from build123d import *

# Parameters (mm, degrees)
F1_DEPTH = 3.81
F2_DEPTH = 25.4
F4_DEPTH = 25.4


with BuildPart() as f1:
    # F0 (on Top) → F1 (new body)
    with BuildSketch(Plane.XY):
        Polygon((6.5642443103, 3.7926732977), (-0.0024292689, 7.5811389783), (-6.5666735793, 3.7884656805), (-6.5642443103, -3.7926732977), (0.0024292689, -7.5811389783), (6.5666735793, -3.7884656805), align=None)
        Polygon((-4.0262038002, 2.3228099792), (-0.00148945, 4.6481997614), (4.0247143502, 2.3253897822), (4.0262038002, -2.3228099792), (0.00148945, -4.6481997614), (-4.0247143502, -2.3253897822), align=None, mode=Mode.SUBTRACT)
    extrude(amount=F1_DEPTH)

    # F2 (add): a face of the model
    f2_faces = [f1.faces().sort_by_distance(p)[0] for p in [
        (3.2845514241, -5.6848023294, 1.905),
    ]]
    extrude(f2_faces, amount=F2_DEPTH)

    # F3 (on face) → F4 (cut)
    with BuildSketch(Plane.XY.offset(3.81)):
        Polygon((3.4240530816, -9.5536917259), (9.0931520865, -16.0562525411), (9.3687364086, -15.8970260939), (6.5666733931, -7.7379561169), (4.9953633304, -8.6458238677), align=None)
        Polygon((9.9074144135, -17.4655531656), (12.7094772591, -25.6246232408), (14.2807875079, -24.7167553825), (10.0452065827, -17.3859399373), align=None)
        Polygon((10.0452065827, -17.3859399373), (14.2807875079, -24.7167553825), (15.8520975706, -23.8088876318), (10.1829987356, -17.3063267185), align=None)
    extrude(amount=-F4_DEPTH, mode=Mode.SUBTRACT)


solid = f1.part
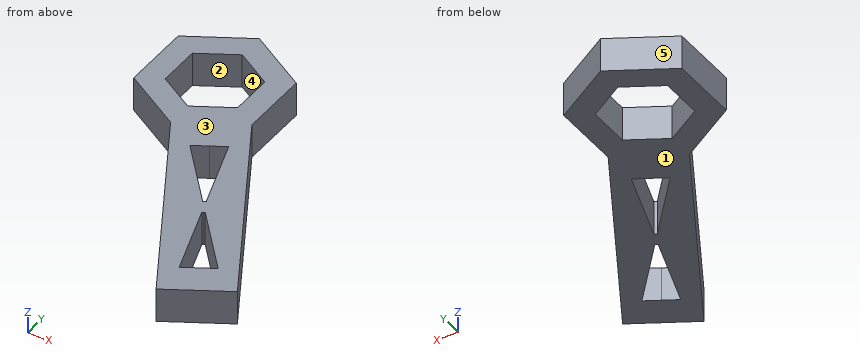
Read the model definition and answer for the solid it produces. Units are mm, in the model's axes. Face numbers are marked on the shaded views. A direction names the side the tool comes from. Give positions to 0.01 mm unless a question says otherwise; leave off trailing zeros. Loops run counter-clockwise (first coordinate to the right, second up) from the corner with the lowest first, then second, coordinate; pieces in that order, holes last. Notation, with made-up numbers: (0.5, 89.25) -> (8.5, 89.25) arc R19 ccw to (8.5, 108.25) -> close; hole circle Ø7 at (62, 81). An arc over 180 degrees is marked (long way). Answer as CSV lines item,"result".
Item 1: Find section B-B on x = -3.5. Give the vertices of the cut face in (y, z).
Returned:
outline,"(-5.56, 0) -> (-2.63, 0) -> (-2.63, 3.81) -> (-5.56, 3.81) -> close; (2.63, 0) -> (5.56, 0) -> (5.56, 3.81) -> (2.63, 3.81) -> close"
Item 2: Find section C-C on z = 2.25. Give the vertices of the cut face in (x, y).
Returned:
outline,"(-6.57, 3.79) -> (-6.56, -3.79) -> (0, -7.58) -> (12.71, -29.57) -> (19.27, -25.78) -> (6.57, -3.79) -> (6.56, 3.79) -> (0, 7.58) -> close; hole (-4.03, 2.32) -> (-4.02, -2.33) -> (0, -4.65) -> (4.03, -2.32) -> (4.02, 2.33) -> (0, 4.65) -> close; hole (3.42, -9.55) -> (9.09, -16.06) -> (9.37, -15.9) -> (6.57, -7.74) -> close; hole (9.91, -17.47) -> (12.71, -25.62) -> (15.85, -23.81) -> (10.18, -17.31) -> close"
Item 3: For the marked faces 1 and 2, determine the directions among +Z, -Z, +X, -X, +Y, -Y from which every point of the face is accessible in a straight line to the end or side of a thin tool.
Returned:
face 1,"-Z, +X, -X, +Y, -Y"
face 2,"+Z, -Z"
Item 4: Consider line 1 (X direction, y = -1, z = 2.45); line 2 (Y direction, x = -3.25, z = 1.95); line 3 (Y direction, x = 15.5, z = 1.95). Determine where each line is inside the solid, lowest interval first. Write a range as [from, to].
Returned:
line 1,"x = [-6.57, -4.03], [4.03, 6.57]"
line 2,"y = [-5.7, -2.77], [2.77, 5.7]"
line 3,"y = [-27.96, -24.01], [-23.41, -19.25]"
Item 5: Determine the mould class of the marked faces 3, 4 and 5 for opening direction Y: +Y half, -Y half, draft (parallel to the pull), parting line (faces both ways), or undercut.
Returned:
face 3,"draft"
face 4,"undercut"
face 5,"+Y half"
Item 6: Each of these flat-tipped pins is pushed along its axis until it touches: pin 1 (1.1 mm diameter, centred on y = -0.5, z = 1, fed in from +X); pin 2 (1.5 mm diameter, centred on y = -24.5, z = 1.5, fed in from -X); pin 3 (2 mm diameter, centred on x = 13, y = -17.5, fed in from -Z). Where does it stop, or does it pass through?
Returned:
pin 1,"stops at x = 6.57"
pin 2,"stops at x = 9.34"
pin 3,"stops at z = 0"
Item 7: Find section A-A on y = -14.5. Give the vertices of the cut face in (x, z).
Returned:
outline,"(4, 0) -> (7.74, 0) -> (7.74, 3.81) -> (4, 3.81) -> close; (8.89, 0) -> (12.76, 0) -> (12.76, 3.81) -> (8.89, 3.81) -> close"
